The listing builds one solid part. Answer for the finished solid, in the listing's coordinates (mm). A direction names the side the tool comes from. Coordinates: 2 decimals unless noted, no trailing zeros. Order: outer loops, then holes, each group sorted by start corner. A loop starts at its lowest first (then second) coordinate and runs counter-clockwise, first axis right, second up. Notation, with made-up numbers: (5, 54) - (59, 54) arc R12 cw to (59, 59) - close; hole circle Ø3 at (13, 50). An arc over 180 degrees is marked (long way). Use a Markdown table: item, result. Add a question column.
Item 1: The part is cut by section A-A, the plane y = 127. Give the vertices of the cut face in (x, z), then the cut area to 3 significant figures.
Item 2: For faces 1 (the flat face through (3.465, 120, 0)), 2 (the flat face through (-3.292, 120, 0)), 3 (the conical face through (-11.65, 101.38, 0.23)), determine the directions among +Z, -Z, +X, -X, +Y, -Y from which every point of the face is accessible in a straight line to the end or side of a thin tool.
Item 3: The mould has two halves that part along Z. Classify faces 4 (the cylindrical face through (-0.33, -5.8, 2.52)), 5 (the cylindrical face through (0.04, 124.48, 0.33)), 6 (the flat face through (-7, 101.6, 0)): released by +Z, released by -Z, zero draft, split by the parting line, or undercut.
Item 4: The part is cut by section C-C, the plane x = 0. Give the vertices of the cut face in (y, z).
Item 5: Find the intervals of material crossed by line 1 along Y through (x, z) = (0.25, 0); line 2 along Z through (x, y) = (-0.5, 127); line 3 along X through (y, z) = (112.5, 3.5), in increasing order.
Item 6: Flat-ended cylindrical pins translate along their axes: P1, Ø8, axis at x = 9, z = 7.5, coming from the +Y side; P2, Ø12, axis at y = 11, z = 8.5, coming from the -X side; P3, Ø12, axis at x = -7, z = 7, coming from the -Y side. Find the tip coordinate at first contact, or state that the pin passes through.
Item 7: The part is cut by section B-B, the plane z = 0. Give the vertices of the cut face in (x, y).
Item 8: The part is cut by section D-D, the plane y = 111.5. Give the vertices of the cut face in (x, z).
Autodesk Inventor part; units mm, degrees
ref_plane "YZ Plane" through (0, 0, 0) normal (1, 0, 0) x (0, 1, 0)
ref_plane "XZ Plane" through (0, 0, 0) normal (0, 1, 0) x (-1, 0, 0)
ref_plane "XY Plane" through (0, 0, 0) normal (0, 0, 1) x (1, 0, 0)
sketch "Sketch1" plane through (0, 0, 0) normal (0, 0, 1) x (1, 0, 0)
  line L0 (0, 0) -> (12.7, 0)
  line L1 (12.7, 0) -> (12.7, 139.7)
  line L2 (12.7, 139.7) -> (0, 139.7)
  line L3 (0, 139.7) -> (0, 0)
  line L4 (0, 0) -> (2.54, 0)
  line L5 (2.54, 0) -> (2.54, -12.7)
  line L6 (2.54, -12.7) -> (0, -12.7)
  line L7 (0, -12.7) -> (0, 0)
  dimension "d0" = 12.7
  dimension "d1" = 139.7
  dimension "d2" = 12.7
  dimension "d3" = 2.54
revolve "Revolution1" add sketch "Sketch1" angle 360 about axis through (0, 139.7, 0) along (0, -1, 0)
sketch "Sketch4" plane through (0, 139.7, 0) normal (0, 1, 0) x (1, 0, 0)
  line L0 (3.175, -12.7) -> (3.175, 12.7)
  line L1 (3.175, 12.7) -> (-3.175, 12.7)
  line L2 (-3.175, 12.7) -> (-3.175, -12.7)
  line L3 (-3.175, -12.7) -> (3.175, -12.7)
  line L4 (3.175, -12.7) -> (-3.175, 12.7) construction
  line L5 (3.175, 12.7) -> (-3.175, -12.7) construction
  point P0 (0, 0)
  dimension "d24" = 6.35
  dimension "d25" = 25.4
sketch "Sketch5" plane through (0, 139.7, 0) normal (0, 1, 0) x (1, 0, 0)
  line L0 (-3.2918, -12.7) -> (-12.7, -12.7)
  line L1 (-12.7, -12.7) -> (-12.7, 12.7)
  line L2 (-12.7, 12.7) -> (-3.2918, 12.7)
  line L3 (-3.2918, 12.7) -> (-3.2918, -12.7)
  line L4 (3.4651, -12.7) -> (12.7, -12.7)
  line L5 (12.7, -12.7) -> (12.7, 12.7)
  line L6 (12.7, 12.7) -> (3.4651, 12.7)
  line L7 (3.4651, 12.7) -> (3.4651, -12.7)
  point P0 (0, 0)
extrude "Extrusion2" cut sketch "Sketch5" against normal blind 38.1
sketch "Sketch6" plane through (3.4651, 139.7, 12.2181) normal (1, 0, 0) x (0, 0, -1)
  line L0 (-0.4819, -139.7) -> (24.9181, -139.7)
  point P0 (12.2181, -139.7)
  point P1 (12.2181, -12.7)
  dimension "d28" = 127
hole "Hole2" at (3.4651, 127, 0) direction (-1, 0, 0) diameter 5.08 end through all
chamfer "Chamfer3" distance 1.27 angle 45 12 edges at (10.1316, 101.6, -7.6578) (10.1316, 101.6, 7.6578) (3.4651, 120.65, -12.2181) (3.4651, 120.65, 12.2181) (3.4651, 139.7, 0) (0.0899, 139.7, -12.6997) (0.0899, 139.7, 12.6997) (-3.2918, 139.7, 0) (-3.2918, 120.65, -12.266) (-3.2918, 120.65, 12.266) (-12.7, 101.6, 0) (-2.54, -12.7, 0)
properties part number "2016.06.13 height guide"
Solution:
| question | item | result |
|---|---|---|
| 1 | outline | (-3.29, -11) - (-2.05, -12.53) arc R12.7 ccw to (2.23, -12.5) - (3.47, -10.95) - (3.47, -2.54) - (-3.29, -2.54) - close; (-3.29, 2.54) - (3.47, 2.54) - (3.47, 10.95) - (2.23, 12.5) arc R12.7 ccw to (-2.05, 12.53) - (-3.29, 11) - close |
| 1 | area | 132 mm2 |
| 2 | face 1 | +Z, -Z, +X, +Y |
| 2 | face 2 | +Z, -Z, -X, +Y |
| 2 | face 3 | -X, +Y |
| 3 | face 4 | split by the parting line |
| 3 | face 5 | undercut |
| 3 | face 6 | zero draft |
| 4 | outline | (-12.7, -1.27) - (-11.43, -2.54) - (0, -2.54) - (0, -12.7) - (138.43, -12.7) - (139.7, -11.43) - (139.7, 11.43) - (138.43, 12.7) - (0, 12.7) - (0, 2.54) - (-11.43, 2.54) - (-12.7, 1.27) - close; hole circle Ø5.08 at (127, 0) |
| 5 | line 1 | y = -12.7 to 124.46, 129.54 to 139.7 |
| 5 | line 2 | z = -12.69 to -2.54, 2.54 to 12.69 |
| 5 | line 3 | x = -3.29 to 3.47 |
| 6 | P1 | stops at y = 101.6 |
| 6 | P2 | stops at x = -12.45 |
| 6 | P3 | stops at y = 0 |
| 7 | outline | (-12.7, 0) - (-2.54, 0) - (-2.54, -11.43) - (-1.27, -12.7) - (1.27, -12.7) - (2.54, -11.43) - (2.54, 0) - (12.7, 0) - (12.7, 100.33) - (11.43, 101.6) - (3.47, 101.6) - (3.47, 124.46) - (-3.29, 124.46) - (-3.29, 101.6) - (-11.43, 101.6) - (-12.7, 100.33) - close; (-3.29, 129.54) - (3.47, 129.54) - (3.47, 138.43) - (2.2, 139.7) - (-2.02, 139.7) - (-3.29, 138.43) - close |
| 8 | outline | (-3.29, -11) - (-2.05, -12.53) arc R12.7 ccw to (2.23, -12.5) - (3.47, -10.95) - (3.47, 10.95) - (2.23, 12.5) arc R12.7 ccw to (-2.05, 12.53) - (-3.29, 11) - close |
